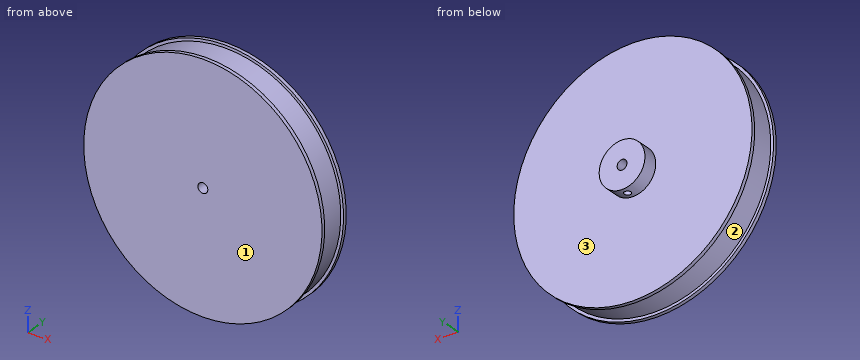
```python
from build123d import *

# Parameters (mm, degrees)
SKETCH1_R           = 32.5
SKETCH1_R_2         = 1.35
BOSS_EXTRUDE1_DEPTH = 9
BOSS_EXTRUDE2_START = 9
SKETCH1_3_R         = 6.25
SKETCH1_3_R_2       = 1.35
BOSS_EXTRUDE2_DEPTH = 4
SKETCH2_W           = 0.75
SKETCH2_H           = 7
SKETCH3_R           = 0.9
CUT_EXTRUDE1_DEPTH  = 10


with BuildPart() as part:
    # Sketch1 → Boss-Extrude1 (new body)
    with BuildSketch(Plane(origin=(0, 0, 0), x_dir=(1, 0, 0), z_dir=(0, 1, 0))):
        with Locations(Location((0, 0, 0), (0, 0, 270))):
            Circle(SKETCH1_R)
        with Locations(Location((0, 0, 0), (0, 0, 270))):
            Circle(SKETCH1_R_2, mode=Mode.SUBTRACT)
    extrude(amount=BOSS_EXTRUDE1_DEPTH)

    # Sketch1<3> → Boss-Extrude2 (add)
    with BuildSketch(Plane(origin=(0, 0, 0), x_dir=(1, 0, 0), z_dir=(0, 1, 0)).offset(BOSS_EXTRUDE2_START)):
        with Locations(Location((0, 0, 0), (0, 0, 270))):
            Circle(SKETCH1_3_R)
        with Locations(Location((0, 0, 0), (0, 0, 270))):
            Circle(SKETCH1_3_R_2, mode=Mode.SUBTRACT)
    extrude(amount=BOSS_EXTRUDE2_DEPTH)

    # Sketch2 → Cut-Revolve1 (revolve, cut)
    with BuildSketch(Plane.XY, mode=Mode.PRIVATE) as cut_revolve1_sk:
        with Locations((32.125, 4.5)):
            Rectangle(SKETCH2_W, SKETCH2_H)
    revolve(cut_revolve1_sk.sketch.rotate(Axis((0, 9, 0), (0, -1, 0)), 90), axis=Axis((0, 9, 0), (0, -1, 0)), mode=Mode.SUBTRACT)

    # Sketch3 → Cut-Extrude1 (cut)
    with BuildSketch(Plane.XY):
        with Locations(Location((0, 11, 0), (0, 0, 90))):
            Circle(SKETCH3_R)
    extrude(amount=-CUT_EXTRUDE1_DEPTH, mode=Mode.SUBTRACT)


solid = part.part
```
CAD build for the part. Positions are in the model's coordinates, mm. Face numbers are marked on the shaded views. Round coordinates to 2 decimals unless told otherwise and drop trailing zeros. Write each loop counter-clockwise with the first axis right and the second up, starting at its lowest first coordinate (ties: lowest second). Pieces come first, ordered by that corner, then holes. Notation, with made-up numbers: (68, -31) - (94, -31) arc R34 ccw to (94, 5) - close; hole circle Ø5 at (69, -20.5). An arc over 180 degrees is marked (long way). Return JSON: item names as keys, results as strings. Group by question number.
Item 1: Probe probe 1 along X at (y, z) = (6.25, 0); probe 2 along Z at (x, y) = (0, 9.75); probe 3 along Y at (x, z) = (-9.5, -7.5). List the from-to ranges inside material, lowest first.
Item 2: Band-saw the part on A-A on x = 0. List the corners of the cut face in (y, z), plus the area to 3 significant figures.
Item 3: Band-saw the part on B-B on z = 0. List the corners of the cut face in (x, y).
Item 4: Band-saw the part on D-D on z = 18. List the corners of the cut face in (x, y), plus the area to 3 significant figures.
Item 5: Flat gauge pins, fed straight in: pin 1 Ø2 at (x, y) = (-2, 1.5) entering from -Z; pin 2 Ø3 at (x, y) = (0, 11) entering from -Z; pin 3 Ø1 at (x, y) = (6.5, 3) entering from +Z; pin 4 Ø1.6 at (x, z) = (0, 0) entering from +Y. Where does each tip first touch, or does it go through?
Item 6: Mould opens along Y. For the marked faces 1, 2 and 3 say: +Y half, -Y half, draft (parallel to the pull), parting line (faces both ways), or undercut.
Item 7: Band-saw the part on C-C on y = 6.5. List the corners of the cut face in (x, z).
Resolved:
{
 "1": {"probe 1": "x = -31.75 to -1.35, 1.35 to 31.75", "probe 2": "z = -6.25 to -1.35, 1.35 to 6.25", "probe 3": "y = 0 to 9"},
 "2": {"outline": "(0, -32.5) - (1, -32.5) - (1, -31.75) - (8, -31.75) - (8, -32.5) - (9, -32.5) - (9, -6.25) - (10.1, -6.25) - (10.1, -1.35) - (0, -1.35) - close; (0, 1.35) - (13, 1.35) - (13, 6.25) - (9, 6.25) - (9, 32.5) - (8, 32.5) - (8, 31.75) - (1, 31.75) - (1, 32.5) - (0, 32.5) - close; (11.9, -6.25) - (13, -6.25) - (13, -1.35) - (11.9, -1.35) - close", "area": "581 mm²"},
 "3": {"outline": "(-32.5, 0) - (-1.35, 0) - (-1.35, 13) - (-6.25, 13) - (-6.25, 9) - (-32.5, 9) - (-32.5, 8) - (-31.75, 8) - (-31.75, 1) - (-32.5, 1) - close; (1.35, 0) - (32.5, 0) - (32.5, 1) - (31.75, 1) - (31.75, 8) - (32.5, 8) - (32.5, 9) - (6.25, 9) - (6.25, 13) - (1.35, 13) - close"},
 "4": {"outline": "(-27.06, 0) - (27.06, 0) - (27.06, 1) - (26.15, 1) - (26.15, 8) - (27.06, 8) - (27.06, 9) - (-27.06, 9) - (-27.06, 8) - (-26.15, 8) - (-26.15, 1) - (-27.06, 1) - close", "area": "474 mm²"},
 "5": {"pin 1": "stops at z = -32.48", "pin 2": "stops at z = -6.25", "pin 3": "stops at z = 31.18", "pin 4": "passes through"},
 "6": {"face 1": "-Y half", "face 2": "undercut", "face 3": "+Y half"},
 "7": {"outline": "circle Ø63.5 at (0, 0); hole circle Ø2.7 at (0, 0)"}
}
